Build history of the part. All positions in model axes, mm. Coordinates: 2 decimals unless noted, no trailing zeros. Write each loop counter-clockwise with the first axis right and the second up, starting at its lowest first coordinate (ties: lowest second). Pieces come first, ordered by that corner, then holes.
Autodesk Inventor part; units mm, degrees
ref_plane "YZ Plane" through (0, 0, 0) normal (1, 0, 0) x (0, 1, 0)
ref_plane "XZ Plane" through (0, 0, 0) normal (0, 1, 0) x (-1, 0, 0)
ref_plane "XY Plane" through (0, 0, 0) normal (0, 0, 1) x (1, 0, 0)
sketch "Sketch1" plane through (0, 0, 0) normal (0, 1, 0) x (-1, 0, 0)
  circle A0 centre (0, 0) radius 8
  arc A1 (-82.4777, 58.296) -> (-82.4777, -58.296) centre (0, 0) ccw construction
  arc A2 (-86.8253, 60.806) -> (-86.8253, -60.806) centre (0, 0) ccw construction
  arc A3 (-2, -11.8322) -> (-2, 11.8322) centre (0, 0) ccw
  line L0 (-2, -11.8322) -> (-89.433, -62.3116)
  arc A4 (-89.433, 62.3116) -> (-89.433, -62.3116) centre (0, 0) ccw
  line L1 (-2, 11.8322) -> (-89.433, 62.3116)
  circle A5 centre (-93.7631, -64.8116) radius 2
  circle A6 centre (-93.7631, 64.8116) radius 2
  circle A7 centre (-114, 0) radius 2
  circle A8 centre (-25, -30.8847) radius 2
  circle A9 centre (-25, 30.8847) radius 2
  circle A10 centre (17, 0) radius 2
  line L2 (10.3923, -6) -> (17, -6)
  arc A11 (17, -6) -> (17, 6) centre (17, 0) ccw
  line L3 (17, 6) -> (10.3923, 6)
  line L4 (-22.3038, -23.5546) -> (-19.8038, -27.8847)
  arc A12 (-30.1962, -33.8847) -> (-19.8038, -27.8847) centre (-25, -30.8847) ccw
  line L5 (-30.1962, -33.8847) -> (-32.6962, -29.5546)
  line L6 (-22.3038, 23.5546) -> (-19.8038, 27.8847)
  arc A13 (-19.8038, 27.8847) -> (-30.1962, 33.8847) centre (-25, 30.8847) ccw
  line L7 (-30.1962, 33.8847) -> (-32.6962, 29.5546)
  line L8 (-92.8025, 57.1726) -> (-96.9102, 59.7032)
  arc A14 (-88.567, 61.8116) -> (-96.9102, 59.7032) centre (-93.7631, 64.8116) ccw
  line L9 (-108.8347, -6) -> (-114, -6)
  arc A15 (-114, 6) -> (-114, -6) centre (-114, 0) ccw
  line L10 (-114, 6) -> (-108.8347, 6)
  line L11 (-92.8025, -57.1726) -> (-96.9102, -59.7032)
  arc A16 (-96.9102, -59.7032) -> (-88.567, -61.8116) centre (-93.7631, -64.8116) ccw
  point P0 (-109, 0)
  point P1 (12, 0)
  dimension "d0" = 16
  dimension "d1" = 101
  dimension "d3" = 12
  dimension "d6" = 60
  dimension "d7" = 2
  dimension "d8" = 5
  dimension "d9" = 3
  dimension "d10" = 4
  dimension "d12" = 5
  dimension "d13" = 5
  dimension "d14" = 5
  dimension "d15" = 5
  dimension "d16" = 5
  dimension "d17" = 5
  dimension "d18" = 25
  dimension "d19" = 6
  dimension "d20" = 6
extrude "Extrusion1" add sketch "Sketch1" along normal blind 6 contours L0 A4 L1 A3
extrude "Extrusion2" add sketch "Sketch1" along normal blind 6 contours A3 L3 A11 L2 | L4 A12 L5 L0 | A16 L11 A4 L0 | L1 L7 A13 L6 | L1 A4 L8 A14 | L9 A15 L10 A4
fillet "Fillet1" radius 8 12 edges at (32.6962, 3, 29.5546) (22.3038, 3, 23.5546) (88.567, 3, 61.8116) (92.8025, 3, 57.1726) (108.8347, 3, -6) (108.8347, 3, 6) (92.8025, 3, -57.1726) (88.567, 3, -61.8116) (32.6962, 3, -29.5546) (22.3038, 3, -23.5546) (2, 3, -11.8322) (-10.3923, 3, 6)
properties part number "RailBaseBottom" material "Polycarbonate, Clear"
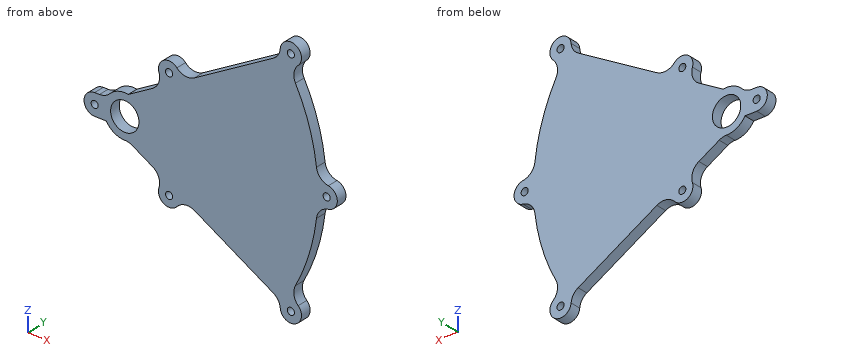
1. Saw through at D-D on x = 61.5. List the corners of the cut face in (y, z), plus the area to 3 significant figures.
Computed values:
outline: (0, -46.18) - (6, -46.18) - (6, 46.18) - (0, 46.18) - close
area: 554 mm2
2. Probe line 1 along Z through (x, y) = (25, 3.65); line 2 along X through (y, z) = (3, -5) (3 decimals); line 3 along Z through (x, y) = (-14, 4.75) (3 decimals). List the from-to ranges inside material, lowest first.
Computed values:
line 1: z = -36.88 to -32.88, -28.88 to 28.88, 32.88 to 36.88
line 2: x = -20.317 to -6.245, 6.245 to 117.317
line 3: z = -6 to 6.005
3. Saw through at A-A on z = 0. List the corners of the cut face in (x, y), plus the area to 3 significant figures.
Computed values:
outline: (-23, 0) - (-19, 0) - (-19, 6) - (-23, 6) - close; (-15, 0) - (-8, 0) - (-8, 6) - (-15, 6) - close; (8, 0) - (112, 0) - (112, 6) - (8, 6) - close; (116, 0) - (120, 0) - (120, 6) - (116, 6) - close
area: 714 mm2
4. Saw through at B-B on x = 25. List the corners of the cut face in (y, z), plus the area to 3 significant figures.
Computed values:
outline: (0, -36.88) - (6, -36.88) - (6, -32.88) - (0, -32.88) - close; (0, -28.88) - (6, -28.88) - (6, 28.88) - (0, 28.88) - close; (0, 32.88) - (6, 32.88) - (6, 36.88) - (0, 36.88) - close
area: 395 mm2
5. Flat gauge pins, fed straight in: pin 1 (5 mm diameter, centred on x = -17, z = 0, fed in from +Y); pin 2 (2 mm diameter, centred on x = -15, y = 3.5, fed in from +Z) (3 decimals); pin 3 (3 mm diameter, centred on x = 93.76, z = -64.81, fed in from -Y); pin 4 (3 mm diameter, centred on y = 2.5, z = 29.5, fed in from -X). Where does each tip first touch, or does it go through?
Computed values:
pin 1: stops at y = 6
pin 2: stops at z = 6.005
pin 3: passes through
pin 4: stops at x = 19
6. Saw through at C-C on y = 1. State how many separate pieces and enclosed holes the cut face has, plus the area to 3 significant figures.
Computed values:
separate pieces: 1
enclosed holes: 7
area: 8,940 mm2
